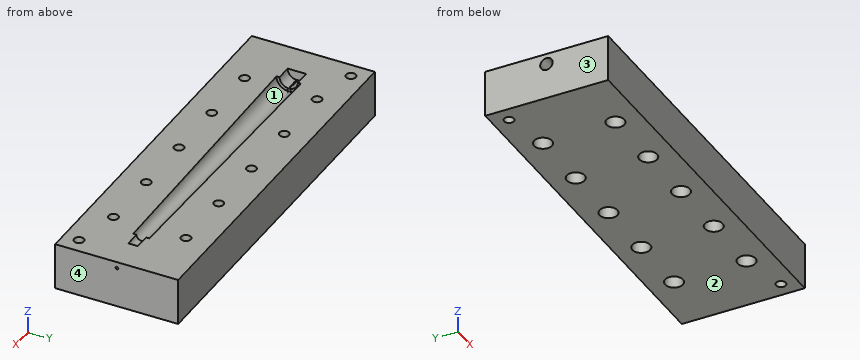
from build123d import *

# Parameters (mm, degrees)
SKIZZE2_W                        = 120
SKIZZE2_H                        = 39.364160046
AUFSATZ_LINEAR_AUSTRAGEN1_DEPTH  = 30
SKIZZE24_R                       = 1.55
SCHNITT_LINEAR_AUSTRAGEN4_DEPTH  = 130.805766806
SKIZZE46_R                       = 2.85
SCHNITT_LINEAR_AUSTRAGEN15_DEPTH = 10
SCHNITT_LINEAR_START             = -5
SCHNITT_LINEAR_AUSTRAGEN25_DEPTH = 2.7
LINEARES_MUSTER1_COUNT           = 5
LINEARES_MUSTER1_PITCH           = 20
SPIEGELN2_COPY_1_SKETCH_R        = 2.85
SPIEGELN2_COPY_1_DEPTH           = 10
SPIEGELN2_COPY_2_SKETCH_R        = 2.85
SPIEGELN2_COPY_2_DEPTH           = 10
SPIEGELN2_COPY_3_SKETCH_R        = 2.85
SPIEGELN2_COPY_3_DEPTH           = 10
SPIEGELN2_COPY_4_SKETCH_R        = 2.85
SPIEGELN2_COPY_4_DEPTH           = 10
SPIEGELN2_START                  = -5
SPIEGELN2_COPY_5_DEPTH           = 2.7
SPIEGELN2_COPY_6_DEPTH           = 2.7
SPIEGELN2_COPY_7_DEPTH           = 2.7
SPIEGELN2_COPY_8_DEPTH           = 2.7
SKIZZE51_R                       = 1.55
SCHNITT_LINEAR_AUSTRAGEN26_DEPTH = 130.805766806
SKIZZE67_R                       = 0.425
SCHNITT_LINEAR_AUSTRAGEN30_DEPTH = 20
SKIZZE70_R                       = 0.5
SCHNITT_LINEAR_AUSTRAGEN37_DEPTH = 16
SKIZZE71_R                       = 2
SCHNITT_LINEAR_AUSTRAGEN38_DEPTH = 6
ABSPALTEN3_START                 = 15
ABSPALTEN3_OUTLINE_W             = 120
ABSPALTEN3_OUTLINE_H             = 39.364160046
ABSPALTEN3_OUTLINE_R             = 1.55
ABSPALTEN3_DEPTH                 = 15


# Read off the part's stored shape, not the designer's step: Abspalten3
with BuildPart() as part:
    # Skizze2 → Aufsatz-Linear austragen1 (new body)
    with BuildSketch(Plane.XY):
        with Locations((60, 19.682080023)):
            Rectangle(SKIZZE2_W, SKIZZE2_H)
    extrude(amount=AUFSATZ_LINEAR_AUSTRAGEN1_DEPTH)

    # Skizze24 → Schnitt-Linear austragen4 (cut, through all)
    with BuildSketch(Plane.XY.offset(30)):
        with Locations((20, 31.364160046)):
            Circle(SKIZZE24_R)
        with Locations((40, 31.364160046)):
            Circle(SKIZZE24_R)
        with Locations((60, 31.364160046)):
            Circle(SKIZZE24_R)
        with Locations((80, 31.364160046)):
            Circle(SKIZZE24_R)
        with Locations((100, 31.364160046)):
            Circle(SKIZZE24_R)
    schnitt_linear_austragen4 = extrude(amount=-SCHNITT_LINEAR_AUSTRAGEN4_DEPTH, mode=Mode.SUBTRACT)

    # Skizze46 → Schnitt-Linear austragen15 (cut)
    with BuildSketch(Plane(origin=(0, 0, 0), x_dir=(-1, 0, 0), z_dir=(0, 0, -1))):
        with Locations((-100, 31.364160046)):
            Circle(SKIZZE46_R)
    schnitt_linear_austragen15 = extrude(amount=-SCHNITT_LINEAR_AUSTRAGEN15_DEPTH, mode=Mode.SUBTRACT)

    # Skizze50 → Schnitt-Linear austragen25 (cut)
    with BuildSketch(Plane.XY.offset(30).offset(SCHNITT_LINEAR_START)):
        Polygon((97.15, 33.009608314), (97.15, 39.364160046), (102.85, 39.364160046), (102.85, 33.009608314), (102.85, 29.718711779), (100, 28.073263512), (97.15, 29.718711779), align=None)
    schnitt_linear_austragen25 = extrude(amount=-SCHNITT_LINEAR_AUSTRAGEN25_DEPTH, mode=Mode.SUBTRACT)

    # Lineares Muster1: Schnitt-Linear austragen15, Schnitt-Linear austragen25 ×5
    with Locations(*[(-i * LINEARES_MUSTER1_PITCH, 0, 0) for i in range(1, LINEARES_MUSTER1_COUNT)]):
        add(schnitt_linear_austragen15, mode=Mode.SUBTRACT)
        add(schnitt_linear_austragen25, mode=Mode.SUBTRACT)

    # Spiegeln2: Schnitt-Linear austragen15, Schnitt-Linear austragen25 across plane
    add(schnitt_linear_austragen15.mirror(Plane.ZX.offset(19.764160046)), mode=Mode.SUBTRACT)
    add(schnitt_linear_austragen25.mirror(Plane.ZX.offset(19.764160046)), mode=Mode.SUBTRACT)

    # Spiegeln2 copy 1 sketch → Spiegeln2 copy 1 (cut)
    with BuildSketch(Plane(origin=(-20, 39.528320093, 0), x_dir=(-1, 0, 0), z_dir=(0, 0, -1))):
        with Locations((-100, -31.364160046)):
            Circle(SPIEGELN2_COPY_1_SKETCH_R)
    extrude(amount=-SPIEGELN2_COPY_1_DEPTH, mode=Mode.SUBTRACT)

    # Spiegeln2 copy 2 sketch → Spiegeln2 copy 2 (cut)
    with BuildSketch(Plane(origin=(-40, 39.528320093, 0), x_dir=(-1, 0, 0), z_dir=(0, 0, -1))):
        with Locations((-100, -31.364160046)):
            Circle(SPIEGELN2_COPY_2_SKETCH_R)
    extrude(amount=-SPIEGELN2_COPY_2_DEPTH, mode=Mode.SUBTRACT)

    # Spiegeln2 copy 3 sketch → Spiegeln2 copy 3 (cut)
    with BuildSketch(Plane(origin=(-60, 39.528320093, 0), x_dir=(-1, 0, 0), z_dir=(0, 0, -1))):
        with Locations((-100, -31.364160046)):
            Circle(SPIEGELN2_COPY_3_SKETCH_R)
    extrude(amount=-SPIEGELN2_COPY_3_DEPTH, mode=Mode.SUBTRACT)

    # Spiegeln2 copy 4 sketch → Spiegeln2 copy 4 (cut)
    with BuildSketch(Plane(origin=(-80, 39.528320093, 0), x_dir=(-1, 0, 0), z_dir=(0, 0, -1))):
        with Locations((-100, -31.364160046)):
            Circle(SPIEGELN2_COPY_4_SKETCH_R)
    extrude(amount=-SPIEGELN2_COPY_4_DEPTH, mode=Mode.SUBTRACT)

    # Spiegeln2 copy 5 sketch → Spiegeln2 copy 5 (cut)
    with BuildSketch(Plane(origin=(-20, 39.528320093, 30), x_dir=(1, 0, 0), z_dir=(0, 0, 1)).offset(SPIEGELN2_START)):
        Polygon((97.15, -33.009608314), (97.15, -39.364160046), (102.85, -39.364160046), (102.85, -33.009608314), (102.85, -29.718711779), (100, -28.073263512), (97.15, -29.718711779), align=None)
    extrude(amount=-SPIEGELN2_COPY_5_DEPTH, mode=Mode.SUBTRACT)

    # Spiegeln2 copy 6 sketch → Spiegeln2 copy 6 (cut)
    with BuildSketch(Plane(origin=(-40, 39.528320093, 30), x_dir=(1, 0, 0), z_dir=(0, 0, 1)).offset(SPIEGELN2_START)):
        Polygon((97.15, -33.009608314), (97.15, -39.364160046), (102.85, -39.364160046), (102.85, -33.009608314), (102.85, -29.718711779), (100, -28.073263512), (97.15, -29.718711779), align=None)
    extrude(amount=-SPIEGELN2_COPY_6_DEPTH, mode=Mode.SUBTRACT)

    # Spiegeln2 copy 7 sketch → Spiegeln2 copy 7 (cut)
    with BuildSketch(Plane(origin=(-60, 39.528320093, 30), x_dir=(1, 0, 0), z_dir=(0, 0, 1)).offset(SPIEGELN2_START)):
        Polygon((97.15, -33.009608314), (97.15, -39.364160046), (102.85, -39.364160046), (102.85, -33.009608314), (102.85, -29.718711779), (100, -28.073263512), (97.15, -29.718711779), align=None)
    extrude(amount=-SPIEGELN2_COPY_7_DEPTH, mode=Mode.SUBTRACT)

    # Spiegeln2 copy 8 sketch → Spiegeln2 copy 8 (cut)
    with BuildSketch(Plane(origin=(-80, 39.528320093, 30), x_dir=(1, 0, 0), z_dir=(0, 0, 1)).offset(SPIEGELN2_START)):
        Polygon((97.15, -33.009608314), (97.15, -39.364160046), (102.85, -39.364160046), (102.85, -33.009608314), (102.85, -29.718711779), (100, -28.073263512), (97.15, -29.718711779), align=None)
    extrude(amount=-SPIEGELN2_COPY_8_DEPTH, mode=Mode.SUBTRACT)

    # Spiegeln3: Schnitt-Linear austragen4 across plane
    add(schnitt_linear_austragen4.mirror(Plane.ZX.offset(19.764160046)), mode=Mode.SUBTRACT)

    # Skizze51 → Schnitt-Linear austragen26 (cut, through all)
    with BuildSketch(Plane.XY.offset(30)):
        with Locations((5, 34.364160046)):
            Circle(SKIZZE51_R)
        with Locations((115, 5)):
            Circle(SKIZZE51_R)
    extrude(amount=-SCHNITT_LINEAR_AUSTRAGEN26_DEPTH, mode=Mode.SUBTRACT)

    # Skizze66 → Schnitt-Rotation5 (revolve, cut)
    with BuildSketch(Plane.XY.offset(15), mode=Mode.PRIVATE) as schnitt_rotation5_sk:
        Polygon((110, 19.682080023), (110, 21.182080023), (10, 22.682080023), (10, 19.682080023), align=None)
        Polygon((105, 19.682080023), (105, 22.257192517), (15, 23.607192517), (15, 19.682080023), align=None)
    revolve(schnitt_rotation5_sk.sketch.rotate(Axis((10, 19.682080023, 15), (1, 0, 0)), 180), axis=Axis((10, 19.682080023, 15), (1, 0, 0)), mode=Mode.SUBTRACT)

    # Skizze67 → Schnitt-Linear austragen30 (cut)
    with BuildSketch(Plane(origin=(120, 0, 0), x_dir=(0, 0, -1), z_dir=(1, 0, 0))):
        with Locations((-17, 19.764160046)):
            Circle(SKIZZE67_R)
    schnitt_linear_austragen30 = extrude(amount=-SCHNITT_LINEAR_AUSTRAGEN30_DEPTH, mode=Mode.SUBTRACT)

    # Spiegeln7: Schnitt-Linear austragen30 across plane
    add(schnitt_linear_austragen30.mirror(Plane.XY.offset(15)), mode=Mode.SUBTRACT)

    # Skizze70 → Schnitt-Linear austragen37 (cut)
    with BuildSketch(Plane.ZY):
        with Locations((11.58373564, 19.764160046)):
            Circle(SKIZZE70_R)
    extrude(amount=-SCHNITT_LINEAR_AUSTRAGEN37_DEPTH, mode=Mode.SUBTRACT)

    # Skizze71 → Schnitt-Linear austragen38 (cut)
    with BuildSketch(Plane.ZY):
        with Locations((11.58373564, 19.764160046)):
            Circle(SKIZZE71_R)
    extrude(amount=-SCHNITT_LINEAR_AUSTRAGEN38_DEPTH, mode=Mode.SUBTRACT)

    # Abspalten3 outline → Abspalten3 (cut)
    with BuildSketch(Plane.XY.offset(ABSPALTEN3_START)):
        with Locations((60, 19.682080023)):
            Rectangle(ABSPALTEN3_OUTLINE_W, ABSPALTEN3_OUTLINE_H)
        with Locations((115, 5)):
            Circle(ABSPALTEN3_OUTLINE_R, mode=Mode.SUBTRACT)
        with Locations((5, 34.364160046)):
            Circle(ABSPALTEN3_OUTLINE_R, mode=Mode.SUBTRACT)
        with Locations((20, 31.364160046)):
            Circle(ABSPALTEN3_OUTLINE_R, mode=Mode.SUBTRACT)
        with Locations((40, 31.364160046)):
            Circle(ABSPALTEN3_OUTLINE_R, mode=Mode.SUBTRACT)
        with Locations((60, 31.364160046)):
            Circle(ABSPALTEN3_OUTLINE_R, mode=Mode.SUBTRACT)
        with Locations((80, 31.364160046)):
            Circle(ABSPALTEN3_OUTLINE_R, mode=Mode.SUBTRACT)
        with Locations((100, 31.364160046)):
            Circle(ABSPALTEN3_OUTLINE_R, mode=Mode.SUBTRACT)
        with Locations((20, 8.164160046)):
            Circle(ABSPALTEN3_OUTLINE_R, mode=Mode.SUBTRACT)
        with Locations((40, 8.164160046)):
            Circle(ABSPALTEN3_OUTLINE_R, mode=Mode.SUBTRACT)
        with Locations((60, 8.164160046)):
            Circle(ABSPALTEN3_OUTLINE_R, mode=Mode.SUBTRACT)
        with Locations((80, 8.164160046)):
            Circle(ABSPALTEN3_OUTLINE_R, mode=Mode.SUBTRACT)
        with Locations((100, 8.164160046)):
            Circle(ABSPALTEN3_OUTLINE_R, mode=Mode.SUBTRACT)
    extrude(amount=ABSPALTEN3_DEPTH, mode=Mode.SUBTRACT)


solid = part.part
CAD build for the part. Positions are in the model's coordinates, mm. Face numbers are marked on the shaded views. Give positions to 0.01 mm unless a question says otherwise; leave off trailing zeros. Order: outer loops, then holes, each group sorted by start corner. A loop starts at its lowest first (then second) coordinate and runs counter-clockwise, first axis right, second up. Notation, with made-up numbers: (51, -17) -> (92, -17) arc R17 cw to (92, -6) -> close; hole circle Ø10 at (73.5, 53.5). An arc over 180 degrees is marked (long way). Return JSON: item names as keys, results as strings.
Q1. Saw through at D-D (x = 60). Write the cut outline in (y, z), then the cut area to 3 significant figures.
Working result:
{"outline": "(0, 0) -> (5.31, 0) -> (5.31, 10) -> (6.61, 10) -> (6.61, 15) -> (0, 15) -> close; (9.71, 10) -> (11.01, 10) -> (11.01, 0) -> (28.51, 0) -> (28.51, 10) -> (29.81, 10) -> (29.81, 15) -> (22.93, 15) arc R3.25 cw to (16.43, 15) -> (9.71, 15) -> close; (32.91, 10) -> (34.21, 10) -> (34.21, 0) -> (39.36, 0) -> (39.36, 15) -> (32.91, 15) -> close", "area": "429 mm²"}
Q2. Saw through at C-C (z = 5.5). Count the separate pieces of the cut face and the enclosed holes in it, then the cut area to 3 significant figures.
Working result:
{"separate pieces": "1", "enclosed holes": "12", "area": "4,450 mm²"}
Q3. Flat gauge pins, fed straight in: pin 1 (5 mm diameter, centred on x = 60, y = 8.16, fed in from -Z); pin 2 (1.2 mm diameter, centred on y = 20.5, z = 11.5, fed in from -X). Where does each tip first touch, or does it go through?
Working result:
{"pin 1": "z = 10", "pin 2": "x = 6"}
Q4. Saw through at B-B (x = 99.5). Write the cut outline in (y, z).
Working result:
{"outline": "(0, 0) -> (5.36, 0) -> (5.36, 10) -> (6.7, 10) -> (6.7, 15) -> (0, 15) -> close; (9.63, 10) -> (10.97, 10) -> (10.97, 0) -> (28.56, 0) -> (28.56, 10) -> (29.9, 10) -> (29.9, 15) -> (22.34, 15) arc R2.66 cw to (17.02, 15) -> (9.63, 15) -> close; (32.83, 10) -> (34.17, 10) -> (34.17, 0) -> (39.36, 0) -> (39.36, 15) -> (32.83, 15) -> close"}
Q5. Drill centre lines: line 1 (X direction, y = 8, z = 11.25); line 2 (Y direction, x = 40, z = 7.25); line 3 (Y direction, x = 80.5, z = 10.25). Where is each one in solid material? Low to high.
Working result:
{"line 1": "0 to 18.46, 21.54 to 38.46, 41.54 to 58.46, 61.54 to 78.46, 81.54 to 98.46, 101.54 to 120", "line 2": "0 to 5.31, 11.01 to 28.51, 34.21 to 39.36", "line 3": "0 to 6.7, 9.63 to 29.9, 32.83 to 39.36"}
Q6. Saw through at A-A (x = 115). Write the cut outline in (y, z) (3 decimals), then the cut area to 3 significant figures.
Working result:
{"outline": "(0, 0) -> (3.45, 0) -> (3.45, 15) -> (0, 15) -> close; (6.55, 0) -> (39.364, 0) -> (39.364, 15) -> (6.55, 15) -> close; hole circle Ø0.85 at (19.764, 13)", "area": "543 mm²"}
Q7. Mould opens along X. For the marked faces 1, 2, 3 and 4 say: pulls with the +X half, pulls with the -X half, needs draft (parallel to the pull), parting line crosses it, or undercut.
Working result:
{"face 1": "undercut", "face 2": "needs draft", "face 3": "pulls with the -X half", "face 4": "pulls with the +X half"}
